```python
from build123d import *

# Parameters (mm, degrees)
SKETCH1_R           = 4.25
BOSS_EXTRUDE1_DEPTH = 5
SKETCH2_R           = 2.1
CUT_EXTRUDE1_DEPTH  = 10


with BuildPart() as part:
    # Sketch1 → Boss-Extrude1 (new body)
    with BuildSketch(Plane.XY):
        Polygon((11.900055679, -27.375), (16.650055679, -22.625), (16.650055679, 22.625), (11.900055679, 27.375), (-7.099944321, 27.375), (-12.099944321, 22.375), (-12.099944321, 15.625), (-16.65, 15.625), (-16.65, -15.625), (-12.099944321, -15.625), (-12.099944321, -22.375), (-7.099944321, -27.375), align=None)
        with Locations((0, -12.485)):
            Circle(SKETCH1_R, mode=Mode.SUBTRACT)
        with Locations(Location((0, 12.485, 0), (0, 0, 180))):
            Circle(SKETCH1_R, mode=Mode.SUBTRACT)
    extrude(amount=BOSS_EXTRUDE1_DEPTH)

    # Sketch2 → Cut-Extrude1 (cut)
    with BuildSketch(Plane(origin=(0, 0, 0), x_dir=(-1, 0, 0), z_dir=(0, 0, -1))):
        with Locations((-13.023685007, -10.001298691)):
            Circle(SKETCH2_R)
        with Locations((-13.023685007, 9.998690221)):
            Circle(SKETCH2_R)
        with Locations((12.976300579, -10.001298691)):
            Circle(SKETCH2_R)
        with Locations((12.976300579, 9.998690221)):
            Circle(SKETCH2_R)
    extrude(amount=-CUT_EXTRUDE1_DEPTH, mode=Mode.SUBTRACT)


solid = part.part
```
Geometry: final body of the model. Coordinates: model frame, mm. A direction names the side the tool comes from. Coordinates: 2 decimals unless noted, no trailing zeros. Order: outer loops, then holes, each group sorted by start corner. A loop starts at its lowest first (then second) coordinate and runs counter-clockwise, first axis right, second up. Notation, with made-up numbers: (-37.75, 59) -> (-24.75, 59) arc R19 cw to (-24.75, 96) -> close; hole circle Ø4 at (-33.75, 85). An arc over 180 degrees is marked (long way). Use CSV: the item, a comma, the result in double quotes.
1) Pin query (flat end, axial travel): pin 1 Ø1.5 at (y, z) = (-18.5, 2.5) entering from -X; pin 2 Ø7.5 at (x, y) = (0, 12.485) entering from -Z; pin 3 Ø3 at (x, z) = (-13, 1.5) entering from +Y; pin 4 Ø2.5 at (x, z) = (-13.5, 3) entering from +Y (3 decimals). Return the tip coordinate at first contact, or that it passes through.
Findings:
pin 1,"stops at x = -12.1"
pin 2,"passes through"
pin 3,"stops at y = 22.97"
pin 4,"stops at y = 15.625"
2) Section B-B on z = 3.7. Output: boundary loops of the cut face in (x, y) (3 decimals), then the cut area to 3 significant figures.
Findings:
outline,"(-16.65, -15.625) -> (-12.1, -15.625) -> (-12.1, -22.375) -> (-7.1, -27.375) -> (11.9, -27.375) -> (16.65, -22.625) -> (16.65, 22.625) -> (11.9, 27.375) -> (-7.1, 27.375) -> (-12.1, 22.375) -> (-12.1, 15.625) -> (-16.65, 15.625) -> close; hole circle Ø4.2 at (-12.976, -10.001); hole circle Ø4.2 at (-12.976, 9.999); hole circle Ø8.5 at (0, -12.485); hole circle Ø8.5 at (0, 12.485); hole circle Ø4.2 at (13.024, -10.001); hole circle Ø4.2 at (13.024, 9.999)"
area,"1,500 mm^2"
3) Access query for faces 1 (the flat face through (-12.1, -19, 2)), 2 (the cylindrical face through (-14.916, 9.194, 2.465)), 3 (the flat face through (-14, 15.625, 2)). Directions: +Z, -Z, +X, -X, +Y, -Y. A direction counts if a zero-diameter tool reaches every point of the face in a straight line with its end or side. Return the directions, or none.
Findings:
face 1,"+Z, -Z, -X, -Y"
face 2,"+Z, -Z"
face 3,"+Z, -Z, -X, +Y"
4) Line query: line 1 (Y direction, x = -13, z = 2.2) (3 decimals); line 2 (Y direction, x = 13, z = 1.4); line 3 (X direction, y = -10, z = 4.35). Output: solid intervals per line, ascending.
Findings:
line 1,"y = -15.625 to -12.101, -7.901 to 7.899, 12.099 to 15.625"
line 2,"y = -26.28 to -12.1, -7.9 to 7.9, 12.1 to 26.28"
line 3,"x = -16.65 to -15.08, -10.88 to -3.45, 3.45 to 10.92, 15.12 to 16.65"
5) Mould query, pull axis Y, two halves, no side actions, for faces 4 (the flat face through (3, 27.375, 2)), 5 (the cylindrical face through (11.084, -10.806, 2.465)), 6 (the flat face through (-12.1, 19, 2)). Classes: +Y half, -Y half, draft (parallel to the pull), parting line (faces both ways), or undercut.
Findings:
face 4,"+Y half"
face 5,"undercut"
face 6,"draft"
6) Section C-C on y = 21. Output: boundary loops of the cut face in (x, z), then the cut area to 3 significant figures.
Findings:
outline,"(-12.1, 0) -> (16.65, 0) -> (16.65, 5) -> (-12.1, 5) -> close"
area,"144 mm^2"
7) Section D-D on x = -14. Output: boundary loops of the cut face in (y, z) (3 decimals).
Findings:
outline,"(-15.625, 0) -> (-11.835, 0) -> (-11.835, 5) -> (-15.625, 5) -> close; (-8.168, 0) -> (8.165, 0) -> (8.165, 5) -> (-8.168, 5) -> close; (11.832, 0) -> (15.625, 0) -> (15.625, 5) -> (11.832, 5) -> close"
8) Section A-A on x = 0. Output: boundary loops of the cut face in (y, z) (3 decimals).
Findings:
outline,"(-27.375, 0) -> (-16.735, 0) -> (-16.735, 5) -> (-27.375, 5) -> close; (-8.235, 0) -> (8.235, 0) -> (8.235, 5) -> (-8.235, 5) -> close; (16.735, 0) -> (27.375, 0) -> (27.375, 5) -> (16.735, 5) -> close"
